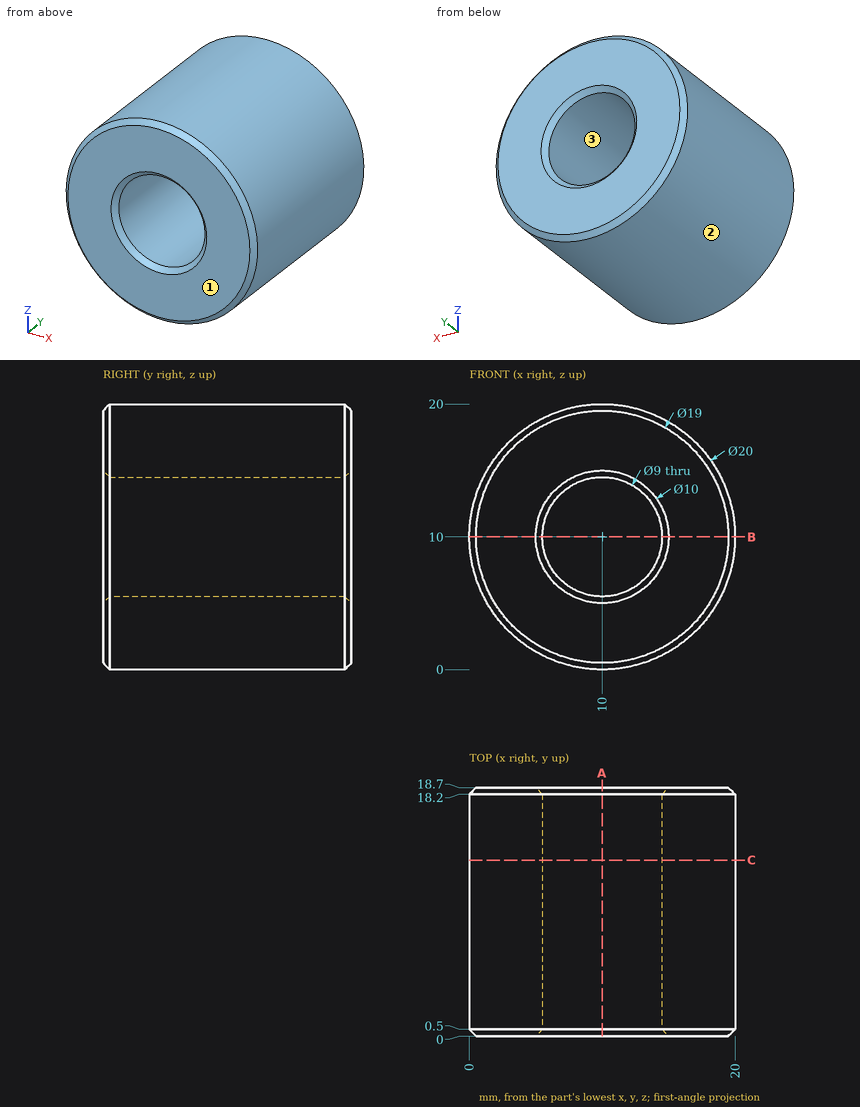
Could you check a few things on this drawing? It's one solid part, dimensions in mm from its lowest x, y, z. Coordinates: 2 decimals unless noted, no trailing zeros. Write each loop counter-clockwise with the first axis right and the second up, starting at its lowest first coordinate (ties: lowest second). Pieces come first, ordered by that corner, then holes.
Q1. Imagine slicing it at A-A, the plane x = 10. List the corners of the cut face in (y, z) for me.
Results found:
outline: (0, 0.5) - (0.5, 0) - (18.2, 0) - (18.7, 0.5) - (18.7, 5) - (18.2, 5.5) - (0.5, 5.5) - (0, 5) - close; (0, 15) - (0.5, 14.5) - (18.2, 14.5) - (18.7, 15) - (18.7, 19.5) - (18.2, 20) - (0.5, 20) - (0, 19.5) - close
Q2. If we mould it in two halves opening along X, with no side actions, what happens to the marked faces 1, 2 and 3? For each: +X half, -X half, draft (parallel to the pull), parting line (faces both ways), or undercut.
Results found:
face 1: draft
face 2: parting line
face 3: undercut
Q3. Please list where these lines run through material, in increasing order: L1, parallel to X at y = 11.25, z = 10; L2, parallel to Z at x = 11.5, y = 11.5; L3, parallel to Z at x = 6.5, y = 15.25.
Results found:
L1: x = 0 to 5.5, 14.5 to 20
L2: z = 0.11 to 5.76, 14.24 to 19.89
L3: z = 0.63 to 7.17, 12.83 to 19.37
Q4. For P1, Ø8, axis at x = 16, y = 3, coming from the -Z side; P2, Ø1, axis at y = 4.5, z = 9, coming from the -X side; P3, Ø5.5, axis at x = 10, z = 10, coming from the -Y side, each with a flat end and sliding along its axis, tell me the tip position at first contact or that it passes through.
Results found:
P1: stops at z = 0.2
P2: stops at x = 0.01
P3: passes through
Q5. Imagine slicing it at B-B, the plane z = 10. List the corners of the cut face in (x, y) for me.
Results found:
outline: (0, 0.5) - (0.5, 0) - (5, 0) - (5.5, 0.5) - (5.5, 18.2) - (5, 18.7) - (0.5, 18.7) - (0, 18.2) - close; (14.5, 0.5) - (15, 0) - (19.5, 0) - (20, 0.5) - (20, 18.2) - (19.5, 18.7) - (15, 18.7) - (14.5, 18.2) - close
Q6. Imagine slicing it at C-C, the plane y = 13.25. List the corners of the cut face in (x, z) for me.
Results found:
outline: circle Ø20 at (10, 10); hole circle Ø9 at (10, 10)
